from build123d import *

# Parameters (mm, degrees)
F0_W      = 1500
F0_H      = 800
F1_DEPTH  = 1200
F2_T      = -40
F4_DEPTH  = 300
F5_W      = 1000
F5_H      = 150
F6_DEPTH  = 300
F7_W      = 50
F7_H      = 575
F8_DEPTH  = 300
F9_W      = 375
F9_H      = 300
F9_R      = 125
F10_DEPTH = 50
F11_R     = 150
F12_DEPTH = 50
F13_W     = 1500
F13_H     = 1200
F14_DEPTH = 50
F15_R     = 160
F15_R_2   = 150
F16_DEPTH = 1250


with BuildPart() as f1:
    # F0 (on Front) → F1 (new body)
    with BuildSketch(Plane.XZ):
        with Locations((750, 400)):
            Rectangle(F0_W, F0_H)
    extrude(amount=F1_DEPTH)

    # F2
    f2_openings = [f1.faces().sort_by_distance(p)[0] for p in [
        (750, -600, 800),
    ]]
    offset(amount=F2_T, openings=f2_openings)

    # F3 (on face) → F4 (join)
    with BuildSketch(Plane(origin=(0, 0, 0), x_dir=(1, 0, 0), z_dir=(0, 0, -1))):
        Polygon((1500, 0), (1500, 50), (50, 50), (50, 1150), (1500, 1150), (1500, 1200), (0, 1200), (0, 0), align=None)
    extrude(amount=F4_DEPTH)

    # F5 (on face) → F6 (join)
    with BuildSketch(Plane(origin=(0, 0, 0), x_dir=(1, 0, 0), z_dir=(0, 0, -1))):
        with Locations((1000, 500)):
            Rectangle(F5_W, F5_H)
    extrude(amount=F6_DEPTH)

    # F7 (on face) → F8 (join)
    with BuildSketch(Plane(origin=(0, 0, 0), x_dir=(1, 0, 0), z_dir=(0, 0, -1))):
        with Locations((1475, 862.5)):
            Rectangle(F7_W, F7_H)
    extrude(amount=F8_DEPTH)

    # F9 (on face) → F10 (join)
    with BuildSketch(Plane.YZ.offset(1500)):
        with Locations((-237.5, -150)):
            Rectangle(F9_W, F9_H)
        with Locations((-237.5, -150)):
            Circle(F9_R, mode=Mode.SUBTRACT)
    extrude(amount=-F10_DEPTH)

    # F11 (on face) → F12 (cut)
    with BuildSketch(Plane(origin=(0, 0, 0), x_dir=(1, 0, 0), z_dir=(0, 0, -1))):
        with Locations((1262.5, 862.5)):
            Circle(F11_R)
    extrude(amount=-F12_DEPTH, mode=Mode.SUBTRACT)

    # F13 (on face) → F14 (join)
    with BuildSketch(Plane(origin=(0, 0, -300), x_dir=(1, 0, 0), z_dir=(0, 0, -1))):
        with Locations((750, 600)):
            Rectangle(F13_W, F13_H)
    extrude(amount=F14_DEPTH)

    # F15 (on face) → F16 (join)
    with BuildSketch(Plane.XY.offset(40)):
        with Locations((1262.5, -862.5)):
            Circle(F15_R)
        with Locations((1262.5, -862.5)):
            Circle(F15_R_2, mode=Mode.SUBTRACT)
    extrude(amount=F16_DEPTH)


solid = f1.part
The model under review builds one solid part; all positions refer to its coordinate system, in mm. A direction names the side the tool comes from. Give positions to 0.01 mm unless a question says otherwise; leave off trailing zeros. Order: outer loops, then holes, each group sorted by start corner. A loop starts at its lowest first (then second) coordinate and runs counter-clockwise, first axis right, second up. Notation, with made-up numbers: M -16,30.5 L 31,30.5 A18 cw 31,38.5 Z; hole C 18.5,-9.75 d3. An arc over 180 degrees is marked long. One line per question, with ' | ' between items. Start each with the question number.
1) Consider section A-A, the plane z = 337.5. Give the boundary of the cut face in (x, y), then the cut area to 3 significant figures.
2) Clearance check with flat-ended pins moving along their axes: P1, Ø6, axis at x = 451.5, y = -777, coming from the +Z side; P2, Ø12, axis at y = -269, z = -154, coming from the +X side. State where each tip first meets the part, or that it passes through.
3) Consider section C-C, the plane x = 201.5. Give the boundary of the cut face in (y, z).
4) Wall thickness on L1, parallel to Y at x = 1262.5, z = 711.5; L2, parallel to X at y = -384, z = 254; L3, parallel to Y at x = 1077, z = 379: over which ranges is each line inside the solid? List them lowest first. Write a range as from..to.
5) Consider section B-B, the plane y = -401. Give the boundary of the cut face in (x, z), then the cut area to 3 significant figures.
6) Mouldability with a two-part tool opening along Y and no side actions: class faces 1 (the face through (0, -592, 233)), 2 (the face through (1151.944, -761.123, 635.97)), 3 (the face through (740, -1200, 233)) as pulls with the +Y half, pulls with the -Y half, needs draft (parallel to the pull), parting line crosses it, or undercut.
7) For faces 4 (the face through (740, -40, 425)), 5 (the face through (1475.35, -264.598, -272.028)), 6 (the face through (760, -50, -148)), 7 (the face through (1309.2, -719.5, 1290)), 8 (the face through (740, -608, -350)), list the 3-axis set-ups (+Z, -Z, +X, -X, +Y, -Y) from which the entire face can be reached by the end or side of a thin tool; tool diameter is ignored.
8) Consider section D-D, the plane x = 581.5. Give the boundary of the cut face in (y, z), then the cut area to 3 significant figures.
Found:
1) outline: M 0,-1200 L 1500,-1200 L 1500,0 L 0,0 Z; C 1262.5,-862.5 d320; hole M 40,-1160 L 1460,-1160 L 1460,-40 L 40,-40 Z; hole C 1262.5,-862.5 d300 | area: 219,000 mm²
2) P1: stops at z = 40 | P2: stops at x = 50
3) outline: M -1200,-350 L 0,-350 L 0,800 L -40,800 L -40,40 L -1160,40 L -1160,800 L -1200,800 Z; hole M -1150,-300 L -50,-300 L -50,0 L -1150,0 Z
4) L1: y = -1200..-1160, -1022.5..-1012.5, -712.5..-702.5, -40..0 | L2: x = 0..40, 1460..1500 | L3: y = -1200..-1160, -40..0
5) outline: M 0,-350 L 1500,-350 L 1500,800 L 1460,800 L 1460,40 L 40,40 L 40,800 L 0,800 Z; hole M 50,-300 L 1450,-300 L 1450,0 L 50,0 Z | area: 226,000 mm²
6) face 1: needs draft | face 2: undercut | face 3: pulls with the -Y half
7) face 4: +Z | face 5: +X | face 6: none | face 7: +Z, +X, -X, +Y, -Y | face 8: -Z, +X, -X, +Y, -Y
8) outline: M -1200,-350 L 0,-350 L 0,800 L -40,800 L -40,40 L -1160,40 L -1160,800 L -1200,800 Z; hole M -1150,-300 L -575,-300 L -575,0 L -1150,0 Z; hole M -425,-300 L -50,-300 L -50,0 L -425,0 Z | area: 244,000 mm²
